```python
from build123d import *

# Parameters (mm, degrees)
ESQUISSE1_W        = 2
ESQUISSE1_H        = 196
BOSS_EXTRU_1_START = -1.5
BOSS_EXTRU_1_DEPTH = 3


# Read off the part's stored shape, not the designer's step: Boss.-Extru.1
with BuildPart() as part:
    # Esquisse1 → R_volution1 (revolve)
    with BuildSketch(Plane.XY):
        with Locations((1, 0)):
            Rectangle(ESQUISSE1_W, ESQUISSE1_H)
    revolve(axis=Axis((0, -98, 0), (0, 1, 0)))

    # Boss.-Extru.1 outline → Boss.-Extru.1 (add)
    with BuildSketch(Plane.XY.offset(BOSS_EXTRU_1_START)):
        with BuildLine():
            Line((2, 88), (4.753939624, 96.450787925))
            ThreePointArc((4.753939624, 96.450787925), (0, 103), (-4.753939624, 96.450787925))
            Line((-4.753939624, 96.450787925), (-2, 88))
            Line((-2, 88), (2, 88))
        make_face()
    boss_extru_1 = extrude(amount=BOSS_EXTRU_1_DEPTH)

    # Esquisse3 → Enl_vement de mati_re-R_volution1 (revolve, cut)
    with BuildSketch(Plane.XY):
        with BuildLine():
            Line((0, 101), (0, 95))
            ThreePointArc((0, 95), (-3, 98), (0, 101))
        make_face()
    enl_vement_de_mati_re_r_volution1 = revolve(axis=Axis((0, 95, 0), (0, 1, 0)), mode=Mode.SUBTRACT)

    # Sym_trie1: Boss.-Extru.1, Enl_vement de mati_re-R_volution1 across plane
    add(boss_extru_1.mirror(Plane.ZX))
    add(enl_vement_de_mati_re_r_volution1.mirror(Plane.ZX), mode=Mode.SUBTRACT)


solid = part.part
```
Read the model definition and answer for the solid it produces. Units are mm, in the model's axes. A direction names the side the tool comes from. Give positions to 0.01 mm unless a question says otherwise; leave off trailing zeros. Write item = value, one per line. Start each with the question number.
Item 1: Find the intervals of material crossed by probe 1 along Y at (x, z) = (-1.25, -0.8); probe 2 along Y at (x, z) = (1.5, 0.6); probe 3 along Z at (x, y) = (-1.5, -69), in increasing order. Write a range as [from, to].
Item 2: A tool of negligible diameter and unlimited length cuts with its end or side. For faces 3 (the flat face through (2, 96, -1.5)), 4 (the flat face through (2, -96, 1.5)), 5 (the cylindrical face through (0, -103, 0)), 6 (the flat face through (2, 96, 1.5)), from which of +Z, -Z, +X, -X, +Y, -Y can it reach the whole face along a straight path? Write none if from no direction.
Item 3: The mould has two halves that part along Y. Classify faces 1 (the flat face through (2, -96, -1.5)), 2 (the cylindrical face through (0, 1, 2)): +Y half, -Y half, draft (parallel to the pull), parting line (faces both ways), or undercut.
Item 4: Each of these flat-tipped pins is pushed along its axis until it touches: P1, Ø3, axis at x = 0, y = 64, coming from the +Z side; P2, Ø5, axis at x = 1.5, y = 93.5, coming from the -Z side; P3, Ø3, axis at y = -35.5, z = 0.5, coming from the -X side. Where does it stop, or does it pass through?
Response:
q1.probe_1 = [-102.84, -100.61], [-95.39, 95.39], [100.61, 102.84]
q1.probe_2 = [-102.77, -100.53], [-95.47, 95.47], [100.53, 102.77]
q1.probe_3 = [-1.32, 1.32]
q2.face_3 = -Z, +Y
q2.face_4 = +Z, -Y
q2.face_5 = +Z, -Z
q2.face_6 = +Z, +Y
q3.face_1 = draft
q3.face_2 = undercut
q4.P1 = 2
q4.P2 = -2
q4.P3 = -2
